Geometry check sheet. Reference: the model listing, model coordinates, mm. Round coordinates to 2 decimals unless told otherwise and drop trailing zeros. Loops run counter-clockwise (first coordinate to the right, second up) from the corner with the lowest first, then second, coordinate; pieces in that order, holes last. Notation, with made-up numbers: M -35,73.5 L -1,73.5 A21 ccw -1,99.5 Z; hole C 75.25,37.25 d1. An arc over 180 degrees is marked long. Write item = value, one per line.
Autodesk Inventor part; units mm, degrees
ref_plane "YZ Plane" through (0, 0, 0) normal (1, 0, 0) x (0, 1, 0)
ref_plane "XZ Plane" through (0, 0, 0) normal (0, 1, 0) x (-1, 0, 0)
ref_plane "XY Plane" through (0, 0, 0) normal (0, 0, 1) x (1, 0, 0)
sketch "Sketch1" plane through (0, 0, 0) normal (0, 0, 1) x (1, 0, 0)
  line L0 (0, 0) -> (183.5, 0)
  line L1 (183.5, 0) -> (183.5, 143)
  line L2 (183.5, 143) -> (0, 143)
  line L3 (0, 143) -> (0, 0)
  dimension "d0" = 183.5
  dimension "d1" = 143
extrude "Extrusion1" add sketch "Sketch1" along normal blind 3
sketch "Sketch3" plane through (0, 0, 3) normal (0, 0, 1) x (1, 0, 0)
  line L0 (0, 0) -> (183.5, 0)
  line L1 (183.5, 0) -> (183.5, 143)
  line L2 (183.5, 143) -> (0, 143)
  line L3 (0, 143) -> (0, 0)
  line L4 (0, 133) -> (183.5, 133) construction
  line L5 (13, 143) -> (13, 0) construction
  line L6 (0, 93) -> (183.5, 93) construction
  line L7 (183.5, 75) -> (0, 75) construction
  line L8 (0, 35) -> (183.5, 35) construction
  line L9 (53, 143) -> (53, 0) construction
  line L10 (130.5, 143) -> (130.5, 0) construction
  line L11 (111.75, 143) -> (111.75, 0) construction
  line L12 (71.75, 143) -> (71.75, 0) construction
  line L13 (170.5, 143) -> (170.5, 0) construction
  line L14 (0, 12) -> (183.5, 12) construction
  point P0 (13, 133)
  point P1 (53, 133)
  point P2 (71.75, 133)
  point P3 (111.75, 133)
  point P4 (130.5, 133)
  point P5 (170.5, 133)
  point P6 (170.5, 93)
  point P7 (130.5, 93)
  point P8 (111.75, 93)
  point P9 (71.75, 93)
  point P10 (53, 93)
  point P11 (13, 93)
  point P12 (53, 35)
  point P13 (53, 75)
  point P14 (13, 75)
  point P15 (13, 35)
  point P16 (130.5, 35)
  point P17 (170.5, 35)
  point P18 (170.5, 75)
  point P19 (130.5, 75)
  point P20 (71.75, 75)
  point P21 (111.75, 75)
  point P22 (111.75, 35)
  point P23 (71.75, 35)
  point P24 (13, 12)
  point P25 (53, 12)
  point P26 (130.5, 12)
  point P27 (170.5, 12)
  dimension "d5" = 40
  dimension "d6" = 40
  dimension "d7" = 40
  dimension "d8" = 40
  dimension "d9" = 40
  dimension "d10" = 13
  dimension "d11" = 13
  dimension "d12" = 10
  dimension "d13" = 18
  dimension "d14" = 18.75
  dimension "d30" = 18.75
  dimension "d40" = 12
hole "Hole1" at (13, 133, 3) at (53, 133, 3) at (71.75, 133, 3) at (111.75, 133, 3) at (130.5, 133, 3) at (170.5, 133, 3) at (170.5, 93, 3) at (130.5, 93, 3) at (111.75, 93, 3) at (71.75, 93, 3) at (53, 93, 3) at (13, 93, 3) at (53, 35, 3) at (53, 75, 3) at (13, 75, 3) at (13, 35, 3) at (130.5, 35, 3) at (170.5, 35, 3) at (170.5, 75, 3) at (130.5, 75, 3) at (71.75, 75, 3) at (111.75, 75, 3) at (71.75, 35, 3) at (111.75, 35, 3) at (13, 12, 3) at (53, 12, 3) at (130.5, 12, 3) at (170.5, 12, 3) direction (0, 0, -1) diameter 4 end through all
sketch "Sketch4" plane through (0, 0, 3) normal (0, 0, 1) x (1, 0, 0)
  circle A0 centre (170.5, 75) radius 2
  circle A1 centre (130.5, 35) radius 2
  circle A2 centre (13, 75) radius 2
  circle A3 centre (53, 35) radius 2
  circle A4 centre (53, 93) radius 2
  circle A5 centre (111.75, 93) radius 2
  circle A6 centre (170.5, 93) radius 2
  circle A7 centre (130.5, 133) radius 2
  circle A8 centre (71.75, 133) radius 2
  circle A9 centre (13, 133) radius 2
  circle A10 centre (53, 133) radius 2
  circle A11 centre (111.75, 133) radius 2
  circle A12 centre (170.5, 133) radius 2
  circle A13 centre (130.5, 93) radius 2
  circle A14 centre (71.75, 93) radius 2
  circle A15 centre (13, 93) radius 2
  circle A16 centre (53, 75) radius 2
  circle A17 centre (13, 35) radius 2
  circle A18 centre (170.5, 35) radius 2
  circle A19 centre (130.5, 75) radius 2
  line L0 (13, 133) -> (53, 93) construction
  line L1 (71.75, 133) -> (111.75, 93) construction
  line L2 (53, 133) -> (13, 93) construction
  line L3 (71.75, 93) -> (111.75, 133) construction
  line L4 (130.5, 133) -> (170.5, 93) construction
  line L5 (170.5, 133) -> (130.5, 93) construction
  line L6 (130.5, 75) -> (170.5, 35) construction
  line L7 (170.5, 75) -> (130.5, 35) construction
  line L8 (13, 75) -> (53, 35) construction
  line L9 (53, 75) -> (13, 35) construction
  circle A20 centre (33, 113) radius 24
  circle A21 centre (91.75, 113) radius 24
  circle A22 centre (150.5, 113) radius 24
  circle A23 centre (150.5, 55) radius 24
  circle A24 centre (33, 55) radius 24
  circle A25 centre (71.75, 35) radius 2
  circle A26 centre (71.75, 75) radius 2
  circle A27 centre (111.75, 75) radius 2
  circle A28 centre (111.75, 35) radius 2
  line L10 (71.75, 75) -> (111.75, 35) construction
  line L11 (111.75, 75) -> (71.75, 35) construction
  circle A29 centre (91.75, 55) radius 24
  dimension "d22" = 48
  dimension "d23" = 48
  dimension "d24" = 48
  dimension "d25" = 48
  dimension "d26" = 48
  dimension "d29" = 48
extrude "Extrusion2" cut sketch "Sketch4" against normal blind 48 contours A20 | A21 | A22 | A23 | A24 | A29
sketch "Sketch5" plane through (0, 0, 3) normal (0, 0, 1) x (1, 0, 0)
  line L0 (0, 0) -> (183.5, 0)
  line L1 (183.5, 0) -> (183.5, 143)
  line L2 (183.5, 143) -> (0, 143)
  line L3 (0, 143) -> (0, 0)
  line L4 (91.75, 143) -> (91.75, 0) construction
  line L5 (85.45, 23.25) -> (98.05, 23.25)
  line L6 (98.05, 23.25) -> (98.05, 12.75)
  line L7 (98.05, 12.75) -> (85.45, 12.75)
  line L8 (85.45, 12.75) -> (85.45, 23.25)
  line L9 (85.45, 23.25) -> (98.05, 12.75) construction
  line L10 (98.05, 23.25) -> (85.45, 12.75) construction
  circle A0 centre (81.87, 18) radius 1.5
  circle A1 centre (101.63, 18) radius 1.5
  line L11 (0, 18) -> (183.5, 18) construction
  point P0 (91.75, 18)
  point P1 (91.75, 18)
  dimension "d31" = 18
  dimension "d32" = 10.5
  dimension "d33" = 12.6
  dimension "d34" = 9.88
  dimension "d35" = 9.88
  dimension "d36" = 3
  dimension "d37" = 3
extrude "Extrusion3" cut sketch "Sketch5" against normal blind 10 contours L5 L6 L7 L8 | A0 | A1
sketch "Sketch6" plane through (0, 0, 3) normal (0, 0, 1) x (1, 0, 0)
  line L0 (0, 0) -> (183.5, 0)
  line L1 (183.5, 0) -> (183.5, 143)
  line L2 (183.5, 143) -> (0, 143)
  line L3 (0, 143) -> (0, 0)
  line L4 (3, 140) -> (180.5, 140)
  line L5 (180.5, 140) -> (180.5, 139)
  line L6 (180.5, 139) -> (3, 139)
  line L7 (3, 139) -> (3, 140)
  line L8 (3, 139) -> (4, 139)
  line L9 (4, 139) -> (4, 5)
  line L10 (4, 5) -> (3, 5)
  line L11 (3, 5) -> (3, 139)
  line L12 (4, 5) -> (179.5, 5)
  line L13 (179.5, 5) -> (179.5, 6)
  line L14 (179.5, 6) -> (4, 6)
  line L15 (4, 6) -> (4, 5)
  line L16 (180.5, 139) -> (179.5, 139)
  line L17 (179.5, 139) -> (179.5, 6)
  line L18 (179.5, 6) -> (180.5, 6)
  line L19 (180.5, 6) -> (180.5, 139)
  line L20 (179.5, 6) -> (180.5, 6)
  line L21 (180.5, 6) -> (180.5, 5)
  line L22 (180.5, 5) -> (179.5, 5)
  line L23 (179.5, 5) -> (179.5, 6)
  dimension "d41" = 1
  dimension "d42" = 1
  dimension "d43" = 1
  dimension "d44" = 1
  dimension "d45" = 3
  dimension "d46" = 3
  dimension "d47" = 3
  dimension "d48" = 5
extrude "Extrusion4" add sketch "Sketch6" along normal blind 1 contours L4 L5 L6 L7 | L6 L9 L10 L11 | L19 L18 L17 L6 | L21 L22 L13 L18 | L14 L13 L12 L9
equation "\"d27\" = d29"
properties part number "plate" material "ABS Plastic"
(1) Sectioned sample at B-B on x = 91.75. Record the cut outline in (y, z).
Result set:
outline = M 0,0 L 12.75,0 L 12.75,3 L 6,3 L 6,4 L 5,4 L 5,3 L 0,3 Z; M 23.25,0 L 31,0 L 31,3 L 23.25,3 Z; M 79,0 L 89,0 L 89,3 L 79,3 Z; M 137,0 L 143,0 L 143,3 L 140,3 L 140,4 L 139,4 L 139,3 L 137,3 Z
(2) Material ranges on line 1 along X through (y, z) = (84.5, 3.4); line 2 along X through (y, z) = (54.5, 2.75); line 3 along X through (y, z) = (12, 1.2), recorded low to high. Write a range as from..to.
Result set:
line_1 = 3..4, 179.5..180.5
line_2 = 0..9.01, 56.99..67.76, 115.74..126.51, 174.49..183.5
line_3 = 0..11, 15..51, 55..128.5, 132.5..168.5, 172.5..183.5
(3) Release check for a two-part mould opening along X. For faces 1 (the cylindrical face through (132.274, 74.077, 1.479)), 2 (the flat face through (70, 73, 0)) record: released by +X, released by -X, zero draft, split by the parting line, or undercut.
Result set:
face_1 = undercut
face_2 = zero draft
(4) Depth check by flat-ended pin: pin 1 Ø10 at (x, y) = (78.5, 84) entering from +Z; pin 2 Ø3.5 at (x, y) = (13, 12) entering from +Z; pin 3 Ø0.9 at (y, z) = (15.5, 1.5) entering from -X; pin 4 Ø0.5 at (x, z) = (61.5, 3.5) entering from -Y. Enter the tip coordinate at first touch or a pass-through.
Result set:
pin_1 = 3
pin_2 = through
pin_3 = 0
pin_4 = 5
(5) Sectioned sample at C-C on z = 1.65. State how many separate pieces and enclosed holes the cut face has, then the cut area to 3 significant figures.
Result set:
separate_pieces = 1
enclosed_holes = 37
area = 14,900 mm2
(6) Sectioned sample at A-A on y = 55. Record the cut outline in (x, z), then the cut area to 4 significant figures.
Result set:
outline = M 0,0 L 9,0 L 9,3 L 4,3 L 4,4 L 3,4 L 3,3 L 0,3 Z; M 57,0 L 67.75,0 L 67.75,3 L 57,3 Z; M 115.75,0 L 126.5,0 L 126.5,3 L 115.75,3 Z; M 174.5,0 L 183.5,0 L 183.5,3 L 180.5,3 L 180.5,4 L 179.5,4 L 179.5,3 L 174.5,3 Z
area = 120.5 mm2
